```python
from build123d import *

# Parameters (mm, degrees)
F0_W         = 44.9817739427
F0_H         = 49.7469753027
F3_DEPTH     = 2
F4_DEPTH     = 12
F2_W         = 37.9821762908
F2_H         = 6.06366992
F5_DEPTH     = 6.6
F6_DEPTH     = 13
F7_R         = 3.5309507028
F7_R_2       = 3.55
F8_DEPTH     = 5
F9_SIZE2     = 12.8533320607
F9_SIZE      = 9
F10_R        = 5
F11_R        = 0.9934278603
F12_DEPTH    = 11
F13_R        = 0.9970874125
F14_DEPTH    = 11
F15_R        = 1.25
F15_R_2      = 1.261860196
F16_DEPTH    = 4
F18_DEPTH    = 29.1
F19_SIZE     = 1.99999
F20_T1_DEPTH = 63.2072532601


# Not quite as in the source:
# - a fillet or chamfer that OpenCascade refuses, or shapes differently, is made with other operations: its cross-section is extruded or revolved along the edge and cut away or added
# - a fillet or chamfer is up to 0.001 mm smaller than in the source, because OpenCascade refuses the exact size


with BuildPart() as f3:
    # F0 (on Top) → F3 (new body)
    with BuildSketch(Plane.XY):
        with Locations((-22.4908869714, 24.8734876513)):
            Rectangle(F0_W, F0_H)
    extrude(amount=-F3_DEPTH)

    # F1 (on face) → F4 (join)
    with BuildSketch(Plane.XY):
        Polygon((-9.6775945276, 22.7995335534), (-9.6775945276, 4.4446666725), (-33.2585461438, 4.2995335534), (-33.2585461438, 22.7995335534), (-38.4990237653, 22.7995335534), (-38.4990237653, 25.7995335534), (-33.2585461438, 25.7995335534), (-33.2585461438, 28.8677942008), (-40.3328314424, 28.8677942008), (-40.3328314424, 18.3987934142), (-34.7744636238, 18.3987934142), (-34.7744636238, 2.8445292264), (-8.1775945276, 2.8445292264), (-8.1775945276, 18.3987934142), (-2.9087525018, 18.3987934142), (-2.9087525018, 28.8677942008), (-9.6775945276, 28.8677942008), (-9.6775945276, 25.7995335534), (-4.7087525018, 25.7995335534), (-4.7087525018, 22.7995335534), align=None)
    extrude(amount=F4_DEPTH)

    # F2 (on Top) → F5 (cut)
    with BuildSketch(Plane.XY):
        with Locations((-21.8701980775, 35.3616550565)):
            Rectangle(F2_W, F2_H)
    extrude(amount=-F5_DEPTH, mode=Mode.SUBTRACT)

    # F1 (on face) → F6 (join)
    with BuildSketch(Plane.XY):
        Polygon((-40.8417806029, 42.3996723965), (-40.8417806029, 40.7995335534), (-2.9438226484, 40.7995335534), (-2.9438226484, 42.3996723965), (-10.0181093439, 42.3996723965), (-10.0181093439, 44.1682427898), (-33.2621894777, 44.1682427898), (-33.2621894777, 42.3996723965), align=None)
    extrude(amount=F6_DEPTH)

    # F7 (on face) → F8 (cut)
    with BuildSketch(Plane(origin=(0, 44.1682427898, 0), x_dir=(-1, 0, 0), z_dir=(0, 1, 0))):
        with Locations((15.6775945276, 6)):
            Circle(F7_R)
        with Locations((27.2585461438, 6)):
            Circle(F7_R_2)
    extrude(amount=-F8_DEPTH, mode=Mode.SUBTRACT)

    # F9
    f9_edges = [f3.edges().sort_by_distance(p)[0] for p in [
        (-40.841781, 41.599603, 13),
        (-2.943823, 41.599603, 13),
    ]]
    f9_side = f3.faces().sort_by_distance((-21.790726, 42.280107, 13))[0]
    chamfer(f9_edges, length=F9_SIZE, length2=F9_SIZE2, reference=f9_side)

    # F10
    f10_edges = [f3.edges().sort_by_distance(p)[0] for p in [
        (-11.943823, 42.483888, 13),
        (-31.841781, 42.483888, 13),
    ]]
    fillet(f10_edges, radius=F10_R)

    # F11 (on face) → F12 (cut)
    with BuildSketch(Plane(origin=(0, 28.8677942008, 0), x_dir=(-1, 0, 0), z_dir=(0, 1, 0))):
        with Locations((6.41001435, 6)):
            Circle(F11_R)
    extrude(amount=-F12_DEPTH, mode=Mode.SUBTRACT)

    # F13 (on face) → F14 (cut)
    with BuildSketch(Plane(origin=(0, 28.8677942008, 0), x_dir=(-1, 0, 0), z_dir=(0, 1, 0))):
        with Locations((36.6457030177, 6)):
            Circle(F13_R)
    extrude(amount=-F14_DEPTH, mode=Mode.SUBTRACT)

    # F15 (on face) → F16 (cut)
    with BuildSketch(Plane(origin=(0, 0, -2), x_dir=(1, 0, 0), z_dir=(0, 0, -1))):
        with Locations((-41.3694195449, -3.6203172058)):
            Circle(F15_R)
        with Locations((-3.4651088063, -3.4644450061)):
            Circle(F15_R_2)
        with Locations((-41.3694195449, -46.0678450763)):
            Circle(F15_R)
        with Locations((-3.4651088063, -46.0678450763)):
            Circle(F15_R)
    extrude(amount=-F16_DEPTH, mode=Mode.SUBTRACT)

    # F17 (on face) → F18 (cut)
    with BuildSketch(Plane(origin=(-34.7744636238, 0, 0), x_dir=(0, -1, 0), z_dir=(-1, 0, 0))):
        Polygon((-2.8445292264, 12), (-18.3987934142, 12), (-4.3348377745, 1.8491647206), (-2.8445292264, 1.8491647206), align=None)
    extrude(amount=-F18_DEPTH, mode=Mode.SUBTRACT)

    # F19 (size 2 in the source; OpenCascade refuses exactly that, so slightly less here)
    f19_edges = [f3.edges().sort_by_distance(p)[0] for p in [
        (-44.981774, 24.873488, -2),
        (0, 24.873488, -2),
    ]]
    chamfer(f19_edges, length=F19_SIZE)

    # F20: chamfer of 2 x 4.289013841 on 2 edges, made by hand

    # F20_s2 → F20_t1 (cut)
    with BuildSketch(Plane.YZ.offset(-54.0945136014)):
        Polygon((2, -2), (0, 2.289013841), (0, -2), align=None)
        Polygon((47.7469753027, -2), (49.7469753027, 2.289013841), (49.7469753027, -2), align=None)
    extrude(amount=F20_T1_DEPTH, mode=Mode.SUBTRACT)


solid = f3.part
```
Geometry: final body of the model. Coordinates: model frame, mm. A direction names the side the tool comes from. Round coordinates to 2 decimals unless told otherwise and drop trailing zeros. Order: outer loops, then holes, each group sorted by start corner. A loop starts at its lowest first (then second) coordinate and runs counter-clockwise, first axis right, second up. Notation, with made-up numbers: (22, 63) - (29, 63) arc R31 ccw to (29, 95) - close; hole circle Ø5 at (74.25, 9.5). An arc over 180 degrees is marked (long way). Use CSV: the item, a comma, the result in double quotes. Start each with the question number.
Q1. Access query for faces 1 (the face through (-9.678, 27, 6)), 2 (the face through (-5.678, 20.63, 6.671)), 3 (the face through (-5, 18.399, 6)), 4 (the face through (-2.909, 24, 6)). Directions: +Z, -Z, +X, -X, +Y, -Y. A direction counts if a zero-diameter tool reaches every point of the face in a straight line with its end or side. Return the directions, or none.
Q2. Material intervals for line 1 along Y through (x, z) = (-6, 1.5); line 2 along X through (y, z) = (23, 1.25); line 3 along X through (y, z) = (15, 8), sorted ascending. Write a range as from..to.
Q3. Section query A-A (z = 1). Return loops of the section in (x, y), and give its area (3 significant figures).
Q4. Section query C-C (x = -17). Return loops of the section in (y, z).
Q5. First-contact query: pin 1 (0.9 mm diameter, centred on y = 27, z = 5, fed in from +X); pin 2 (3.5 mm diameter, centred on x = -7, z = 5, fed in from +Y); pin 3 (2.5 mm diameter, centred on x = -6.5, z = 8, fed in from -Y); pin 4 (3.5 mm diameter, centred on x = -3.47, y = 3.46, fed in from -Z). Flat tips, straight axial feed; report the tip coordinate or a pass-through.
Q6. Mould query, pull axis X, two halves, no side actions, for faces 5 (the face through (-34.03, 11.47, 7)), 6 (the face through (-43.996, 24.54, -0.986)), 7 (the face through (-4.709, 24, 6)), 8 (the face through (-5.678, 27.355, 6.671)). Classes: +X half, -X half, draft (parallel to the pull), parting line (faces both ways), or undercut.
Result set:
1,face 1,"+Z"
1,face 2,"-Y"
1,face 3,"+Z, +X, -Y"
1,face 4,"+Z, +X, +Y, -Y"
2,line 1,"y = 18.4..22.8, 25.8..28.87, 40.8..42.4"
2,line 2,"x = -40.33..-38.5, -4.71..-2.91"
2,line 3,"x = -34.77..-33.26, -9.68..-8.18"
3,outline,"(-40.33, 18.4) - (-34.77, 18.4) - (-34.77, 2.84) - (-8.18, 2.84) - (-8.18, 18.4) - (-2.91, 18.4) - (-2.91, 28.87) - (-9.68, 28.87) - (-9.68, 25.8) - (-4.71, 25.8) - (-4.71, 22.8) - (-9.68, 22.8) - (-9.68, 4.44) - (-33.26, 4.3) - (-33.26, 22.8) - (-38.5, 22.8) - (-38.5, 25.8) - (-33.26, 25.8) - (-33.26, 28.87) - (-40.33, 28.87) - close; (-40.24, 40.8) - (-3.54, 40.8) - (-3.54, 42.4) - (-10.02, 42.4) - (-10.02, 44.17) - (-33.26, 44.17) - (-33.26, 42.4) - (-40.24, 42.4) - close"
3,area,"297 mm2"
4,outline,"(1.07, 0) - (2, -2) - (32.33, -2) - (32.33, 0) - (4.4, 0) - (4.4, 1.9) - (4.33, 1.85) - (2.84, 1.85) - (2.84, 0) - close; (38.39, -2) - (47.75, -2) - (48.68, 0) - (44.17, 0) - (44.17, 2.73) - (40.8, 2.73) - (40.8, 0) - (38.39, 0) - close; (40.8, 9.27) - (44.17, 9.27) - (44.17, 13) - (40.8, 13) - close"
5,pin 1,"stops at x = -2.91"
5,pin 2,"stops at y = 42.4"
5,pin 3,"stops at y = 18.4"
5,pin 4,"stops at z = -2"
6,face 5,"draft"
6,face 6,"-X half"
6,face 7,"undercut"
6,face 8,"undercut"
